```python
from build123d import *

# Parameters (mm, degrees)
SKETCH_1_W          = 25
SKETCH_1_H          = 25
SKETCH_1_R          = 1.75
EXTRUDE_1_DEPTH     = 5
SKETCH_2_R          = 7.905
CUT_EXTRUDE_1_DEPTH = 5
SKETCH_3_R          = 10.5
SKETCH_3_R_2        = 7.905
EXTRUDE_2_DEPTH     = 20


with BuildPart() as part:
    # 草图1 → 凸台-拉伸1 (new body)
    with BuildSketch(Plane.XY):
        Rectangle(SKETCH_1_W, SKETCH_1_H)
        with Locations((-9.5, 9.5)):
            Circle(SKETCH_1_R, mode=Mode.SUBTRACT)
        with Locations((-9.5, -9.5)):
            Circle(SKETCH_1_R, mode=Mode.SUBTRACT)
        with Locations((9.5, -9.5)):
            Circle(SKETCH_1_R, mode=Mode.SUBTRACT)
        with Locations((9.5, 9.5)):
            Circle(SKETCH_1_R, mode=Mode.SUBTRACT)
    extrude(amount=EXTRUDE_1_DEPTH)

    # 草图2 → 切除-拉伸1 (cut)
    with BuildSketch(Plane.XY.offset(5)):
        Circle(SKETCH_2_R)
    extrude(amount=-CUT_EXTRUDE_1_DEPTH, mode=Mode.SUBTRACT)

    # 草图3 → 凸台-拉伸2 (add)
    with BuildSketch(Plane.XY.offset(5)):
        Circle(SKETCH_3_R)
        Circle(SKETCH_3_R_2, mode=Mode.SUBTRACT)
    extrude(amount=EXTRUDE_2_DEPTH)


solid = part.part
```
Here's how the part is built. I have some questions about the finished solid (model axes, mm). A direction names the side the tool comes from. Round coordinates to 2 decimals unless told otherwise and drop trailing zeros. Loops run counter-clockwise (first coordinate to the right, second up) from the corner with the lowest first, then second, coordinate; pieces in that order, holes last.
1. If I drill on probe 1 along Y at (x, z) = (9.5, 3.3); probe 2 along Y at (x, z) = (-1.25, 14.75); probe 3 along Y at (x, z) = (-6.5, 19), over which ranges is the centre line in solid material (lowest first)?
Answers:
probe 1: y = -12.5 to -11.25, -7.75 to 7.75, 11.25 to 12.5
probe 2: y = -10.43 to -7.81, 7.81 to 10.43
probe 3: y = -8.25 to -4.5, 4.5 to 8.25
2. Suppose I cut it at C-C, the plane x = 9.5. Please give me the cut outline in (y, z).
Answers:
outline: (-12.5, 0) - (-11.25, 0) - (-11.25, 5) - (-12.5, 5) - close; (-7.75, 0) - (7.75, 0) - (7.75, 5) - (4.47, 5) - (4.47, 25) - (-4.47, 25) - (-4.47, 5) - (-7.75, 5) - close; (11.25, 0) - (12.5, 0) - (12.5, 5) - (11.25, 5) - close
3. Suppose I cut it at D-D, the plane x = 3.25. Please give me the cut outline in (y, z), and give its area (3 significant figures).
Answers:
outline: (-12.5, 0) - (-7.21, 0) - (-7.21, 25) - (-9.98, 25) - (-9.98, 5) - (-12.5, 5) - close; (7.21, 0) - (12.5, 0) - (12.5, 5) - (9.98, 5) - (9.98, 25) - (7.21, 25) - close
area: 164 mm2
4. Suppose I cut it at A-A, the plane y = 0. Please give me the cut outline in (x, z) (3 decimals).
Answers:
outline: (-12.5, 0) - (-7.905, 0) - (-7.905, 25) - (-10.5, 25) - (-10.5, 5) - (-12.5, 5) - close; (7.905, 0) - (12.5, 0) - (12.5, 5) - (10.5, 5) - (10.5, 25) - (7.905, 25) - close
5. Suppose I cut it at B-B, the plane z = 1.5. Please give me the cut outline in (x, y) (3 decimals).
Answers:
outline: (-12.5, -12.5) - (12.5, -12.5) - (12.5, 12.5) - (-12.5, 12.5) - close; hole circle Ø3.5 at (-9.5, -9.5); hole circle Ø3.5 at (-9.5, 9.5); hole circle Ø15.81 at (0, 0); hole circle Ø3.5 at (9.5, -9.5); hole circle Ø3.5 at (9.5, 9.5)
6. Thinking about a two-plate mould opening in Y: for faces 3 (the face through (0, -12.5, 2)), 4 (the face through (-1.029, 7.838, 12.325)), 5 (the face through (0, -11, 5)), which applies, released by +Y, released by -Y, zero draft, split by the parting line, or undercut?
Answers:
face 3: released by -Y
face 4: undercut
face 5: zero draft
7. Will these pins go through, and if not, where does the flat tip stop? pin 1 (1.5 mm diameter, centred on x = 0.5, z = 20.5, fed in from -Y); pin 2 (1 mm diameter, centred on x = 1.5, y = -6, fed in from -Z) (1 decimal); pin 3 (12 mm diameter, centred on y = 0, z = 18, fed in from -X); pin 4 (10 mm diameter, centred on y = -9.5, z = 17.5, fed in from +X).
Answers:
pin 1: stops at y = -10.5
pin 2: passes through
pin 3: stops at x = -10.5
pin 4: stops at x = 9.49
8. For faces 1 (the face through (10.4, -8, 2.5)), 2 (the face through (10, 3.2, 14.9)), which set-ups out of +Z, -Z, +X, -X, +Y, -Y let a thin tool reach every point of the face, with its end or its side?
Answers:
face 1: +Z, -Z
face 2: +Z
